Read the model definition and answer for the solid it produces. Units are mm, in the model's axes. A direction names the side the tool comes from. Coordinates: 2 decimals unless noted, no trailing zeros. Loops run counter-clockwise (first coordinate to the right, second up) from the corner with the lowest first, then second, coordinate; pieces in that order, holes last. Notation, with made-up numbers: (-38.75, 51.25) -> (-22.75, 51.25) arc R30 ccw to (-22.75, 89.25) -> close; hole circle Ø2 at (-40, 43.5). An arc over 180 degrees is marked (long way). Answer as a JSON object with one key per item and string values. Group by question number.
Q1. For faces 1 (the cylindrical face through (-11.81, 3.72, 10.13)), 2 (the flat face through (0, 0, -120.65)), 3 (the flat face through (0, -6, -19.05)), determine the directions among +Z, -Z, +X, -X, +Y, -Y from which every point of the face is accessible in a straight line to the end or side of a thin tool.
Q2. Each of these flat-tipped pins is pushed along its axis until it touches: P1, Ø12, axis at x = 4.5, z = -84.5, coming from the +Y side; P2, Ø5, axis at y = -5.5, z = -76.5, coming from the +X side; P3, Ø6, axis at x = -17.5, y = -14.5, coming from the +Z side. Where does it stop, or does it pass through?
Q3. Determine the mould class of faces 4 (the flat face through (-11.23, -5.59, 7.938)), 5 (the flat face through (12.4, -4, 0)), 6 (the cylindrical face through (-1.204, -5.424, -69.139)) for opening direction Y: released by +Y, released by -Y, zero draft, split by the parting line, or undercut.
Q4. The part is cut by section A-A on z = -46. Write down the section's boundary in (x, y).
Q5. Straight lines are drawn through the part: line 1 along Y through (x, z) = (0, 3.55); line 2 along Y through (x, z) = (0, 9.2); line 3 along Z through (x, y) = (9, -7). For each, find the intervals that lie inside material, in ascending order. Write a range as [from, to].
Autodesk Inventor part; units mm, degrees
ref_plane "Work Plane1" through (0, 0, 6.35) normal (0, 0, -1) x (-1, 0, 0)
ref_plane "YZ Plane" through (0, 0, 0) normal (1, 0, 0) x (0, 1, 0)
ref_plane "XZ Plane" through (0, 0, 0) normal (0, 1, 0) x (-1, 0, 0)
sketch "Sketch1" plane through (0, 0, 0) normal (0, 0, 1) x (1, 0, 0)
  circle A0 centre (0, 0) radius 25.4
  circle A1 centre (0, 0) radius 12.7
  dimension "d0" = 50.8
  dimension "d1" = 25.4
extrude "Extrusion1" add sketch "Sketch1" along normal blind 12.7
fillet "Fillet1" radius 6.35 2 edges at (-25.4, 0, 12.7) (-25.4, 0, 0)
sketch "Sketch2" plane through (0, 0, 12.7) normal (0, 0, 1) x (1, 0, 0)
  circle A0 centre (0, 0) radius 12.7
  circle A1 centre (0, 0) radius 19.05
  circle A2 centre (0, 0) radius 5.5563
  dimension "d5" = 11.1125
extrude "Extrusion2" add sketch "Sketch2" against normal blind 133.35 contours A2
ref_plane "Work Plane1" through (0, 0, 6.35) normal (0, 0, -1) x (-1, 0, 0)
sketch "Sketch3" plane through (0, 0, 6.35) normal (0, 0, -1) x (-1, 0, 0)
  circle A0 centre (0, 0) radius 12.3825
  circle A1 centre (0, 0) radius 5.7531
  dimension "d8" = 24.765
  dimension "d9" = 11.5062
extrude "Extrusion3" add sketch "Sketch3" along normal mid plane 12.065
sketch "Sketch4" plane through (0, 0, 6.35) normal (0, 0, -1) x (-1, 0, 0)
  circle A0 centre (0, 0) radius 6.35
  dimension "d12" = 12.7
extrude "Extrusion4" add sketch "Sketch4" along normal blind 25.4
sketch "Sketch5" plane through (0, 0, 6.35) normal (0, 0, -1) x (-1, 0, 0)
  circle A0 centre (0, 0) radius 19.05
  dimension "d15" = 38.1
extrude "Extrusion5" add sketch "Sketch5" along normal mid plane 3.175
properties part number "2in roller" material "Steel, Alloy"
Final values:
{
 "1": {"face 1": "+Z", "face 2": "-Z, +X, -X, +Y, -Y", "face 3": "-Z"},
 "2": {"P1": "stops at y = 5.56", "P2": "stops at x = 4.68", "P3": "stops at z = 12.66"},
 "3": {"face 4": "undercut", "face 5": "zero draft", "face 6": "split by the parting line"},
 "4": {"outline": "circle Ø11.11 at (0, 0)"},
 "5": {"line 1": "y = [-24.75, -12.7], [-12.38, 12.38], [12.7, 24.75]", "line 2": "y = [-24.72, -12.7], [-12.38, -5.75], [-5.56, 5.56], [5.75, 12.38], [12.7, 24.72]", "line 3": "z = [0.32, 12.38]"}
}
